Geometry check sheet. Reference: the model listing, model coordinates, mm. A direction names the side the tool comes from. Give positions to 0.01 mm unless a question says otherwise; leave off trailing zeros. Write each loop counter-clockwise with the first axis right and the second up, starting at its lowest first coordinate (ties: lowest second). Pieces come first, ordered by that corner, then holes. Notation, with made-up numbers: (-4.5, -13.75) - (26.5, -13.75) arc R13 cw to (26.5, -7.75) - close; hole circle Ø7 at (18, 76). An arc over 180 degrees is marked (long way). Use a Markdown table: item, result.
```python
from build123d import *

# Parameters (mm, degrees)
SKETCH1_W                    = 86
SKETCH1_H                    = 90
BASE_FLANGE1_DEPTH           = 2
EDGE_FLANGE1_STRIP_W         = 9.4732
EDGE_FLANGE1_STRIP_H         = 2
EDGE_FLANGE1_STRIP_CUT_DEPTH = 90
EDGE_FLANGE1_DEPTH           = 90
EDGE_FLANGE2_STRIP_W         = 9.4732
EDGE_FLANGE2_STRIP_H         = 2
EDGE_FLANGE2_STRIP_CUT_DEPTH = 90
EDGE_FLANGE2_DEPTH           = 90
SKETCH13_W                   = 25
SKETCH13_H                   = 22.2634
CUT_EXTRUDE1_DEPTH           = 127.980922721
SKETCH15_R                   = 5
CUT_EXTRUDE2_DEPTH           = 127.980922721


# Sheet-metal steps are written as plain solids
with BuildPart() as part:
    # Sketch1 → Base-Flange1 (new body)
    with BuildSketch(Plane(origin=(0, 0, 0), x_dir=(1, 0, 0), z_dir=(0, 1, 0))):
        with Locations((47.016874378, 45.0175246)):
            Rectangle(SKETCH1_W, SKETCH1_H)
    extrude(amount=-BASE_FLANGE1_DEPTH)

    # Edge-Flange1 strip (across the edge) → Edge-Flange1 strip cut (cut)
    with BuildSketch(Plane(origin=(90.016874378, -2, -90.0175246), x_dir=(-1, 0, 0), z_dir=(0, 0, 1))):
        with Locations((-2, -1)):
            Rectangle(EDGE_FLANGE1_STRIP_W, EDGE_FLANGE1_STRIP_H)
    extrude(amount=EDGE_FLANGE1_STRIP_CUT_DEPTH, mode=Mode.SUBTRACT)

    # Edge-Flange1 section (across the edge) → Edge-Flange1 (add)
    with BuildSketch(Plane(origin=(90.016874378, -2, -90.0175246), x_dir=(-1, 0, 0), z_dir=(0, 0, 1))):
        with BuildLine():
            Line((0, 0.7366), (0, 23))
            Line((0, 23), (2, 23))
            Line((2, 23), (2, 0.7366))
            ThreePointArc((2, 0.7366), (2.215745145, 0.215745145), (2.7366, 0))
            Line((2.7366, 0), (2.7366, -2))
            ThreePointArc((2.7366, -2), (0.801531583, -1.198468417), (0, 0.7366))
        make_face()
    extrude(amount=EDGE_FLANGE1_DEPTH)

    # Edge-Flange2 strip (across the edge) → Edge-Flange2 strip cut (cut)
    with BuildSketch(Plane(origin=(4.016874378, -2, -0.0175246), x_dir=(1, 0, 0), z_dir=(0, 0, -1))):
        with Locations((-2, -1)):
            Rectangle(EDGE_FLANGE2_STRIP_W, EDGE_FLANGE2_STRIP_H)
    extrude(amount=EDGE_FLANGE2_STRIP_CUT_DEPTH, mode=Mode.SUBTRACT)

    # Edge-Flange2 section (across the edge) → Edge-Flange2 (add)
    with BuildSketch(Plane(origin=(4.016874378, -2, -0.0175246), x_dir=(1, 0, 0), z_dir=(0, 0, -1))):
        with BuildLine():
            Line((0, 0.7366), (0, 23))
            Line((0, 23), (2, 23))
            Line((2, 23), (2, 0.7366))
            ThreePointArc((2, 0.7366), (2.215745145, 0.215745145), (2.7366, 0))
            Line((2.7366, 0), (2.7366, -2))
            ThreePointArc((2.7366, -2), (0.801531583, -1.198468417), (0, 0.7366))
        make_face()
    extrude(amount=EDGE_FLANGE2_DEPTH)

    # Sketch13 → Cut-Extrude1 (cut, through all)
    with BuildSketch(Plane(origin=(90.016874378, 0, 0), x_dir=(0, 0, -1), z_dir=(1, 0, 0))):
        with Locations((25.5175246, -13.8683)):
            Rectangle(SKETCH13_W, SKETCH13_H)
    extrude(amount=-CUT_EXTRUDE1_DEPTH, mode=Mode.SUBTRACT)

    # Sketch15 → Cut-Extrude2 (cut, through all)
    with BuildSketch(Plane.ZY.offset(-4.016874378)):
        with Locations(Location((-75.0175246, -17.7366, 0), (0, 0, 270))):
            Circle(SKETCH15_R)
    extrude(amount=-CUT_EXTRUDE2_DEPTH, mode=Mode.SUBTRACT)


solid = part.part
```
1) Depth check by flat-ended pin: P1, Ø8, axis at y = -17.74, z = -75.02, coming from the +X side; P2, Ø0.6, axis at x = 5, z = -23, coming from the -Y side. Enter the tip coordinate at first touch or a pass-through.
Working result:
| item | result |
|---|---|
| P1 | passes through |
| P2 | stops at y = -2.74 |
2) Section check D-D on x = 36.5. Record the boundary of the cut face in (y, z).
Working result:
| item | result |
|---|---|
| outline | (-2, -90.02) - (0, -90.02) - (0, -0.02) - (-2, -0.02) - close |
3) Mould release check, pull along X, two halves, no side actions. Record for faces 3 (the flat face through (4.017, -14, -64)), 4 (the flat face through (90.017, -14, -64)), 5 (the flat face through (88.017, -14, -7)), 6 (the flat face through (89, -14, -13.018)): pulls with the +X half, pulls with the -X half, needs draft (parallel to the pull), parting line crosses it, or undercut.
Working result:
| item | result |
|---|---|
| face 3 | pulls with the -X half |
| face 4 | pulls with the +X half |
| face 5 | undercut |
| face 6 | needs draft |
4) Section check B-B on z = -64.5. Record the boundary of the cut face in (x, y), then the cut area to 3 significant figures.
Working result:
| item | result |
|---|---|
| outline | (4.02, -25) - (6.02, -25) - (6.02, -2.74) arc R0.74 cw to (6.75, -2) - (87.28, -2) arc R0.74 cw to (88.02, -2.74) - (88.02, -25) - (90.02, -25) - (90.02, -2.74) arc R2.74 ccw to (87.28, 0) - (6.75, 0) arc R2.74 ccw to (4.02, -2.74) - close |
| area | 261 mm² |
5) Section check C-C on y = -18.75. Record the boundary of the cut face in (x, z).
Working result:
| item | result |
|---|---|
| outline | (4.02, -90.02) - (6.02, -90.02) - (6.02, -79.91) - (4.02, -79.91) - close; (4.02, -70.12) - (6.02, -70.12) - (6.02, -38.02) - (4.02, -38.02) - close; (4.02, -13.02) - (6.02, -13.02) - (6.02, -0.02) - (4.02, -0.02) - close; (88.02, -90.02) - (90.02, -90.02) - (90.02, -79.91) - (88.02, -79.91) - close; (88.02, -70.12) - (90.02, -70.12) - (90.02, -38.02) - (88.02, -38.02) - close; (88.02, -13.02) - (90.02, -13.02) - (90.02, -0.02) - (88.02, -0.02) - close |
6) Section check A-A on y = -8.75. Record the boundary of the cut face in (x, z).
Working result:
| item | result |
|---|---|
| outline | (4.02, -90.02) - (6.02, -90.02) - (6.02, -38.02) - (4.02, -38.02) - close; (4.02, -13.02) - (6.02, -13.02) - (6.02, -0.02) - (4.02, -0.02) - close; (88.02, -90.02) - (90.02, -90.02) - (90.02, -38.02) - (88.02, -38.02) - close; (88.02, -13.02) - (90.02, -13.02) - (90.02, -0.02) - (88.02, -0.02) - close |
7) Set-up check for faces 1 (the flat face through (5, -2.737, -25)), 2 (the cylindrical face through (89.194, -0.78, -45.648)): record each of +Z, -Z, +X, -X, +Y, -Y from which the full face is reachable in a straight line by a thin tool's end or side.
Working result:
| item | result |
|---|---|
| face 1 | +X, -X, -Y |
| face 2 | +Z, -Z, +X, +Y |
8) Material ranges on L1, parallel to X at y = -5.75, z = -51.5; L2, parallel to Y at x = 49, z = -6.5; L3, parallel to X at y = -2.5, z = -9, recorded low to high. Write a range as from..to.
Working result:
| item | result |
|---|---|
| L1 | x = 4.02..6.02, 88.02..90.02 |
| L2 | y = -2..0 |
| L3 | x = 4.03..6.06, 87.98..90.01 |
